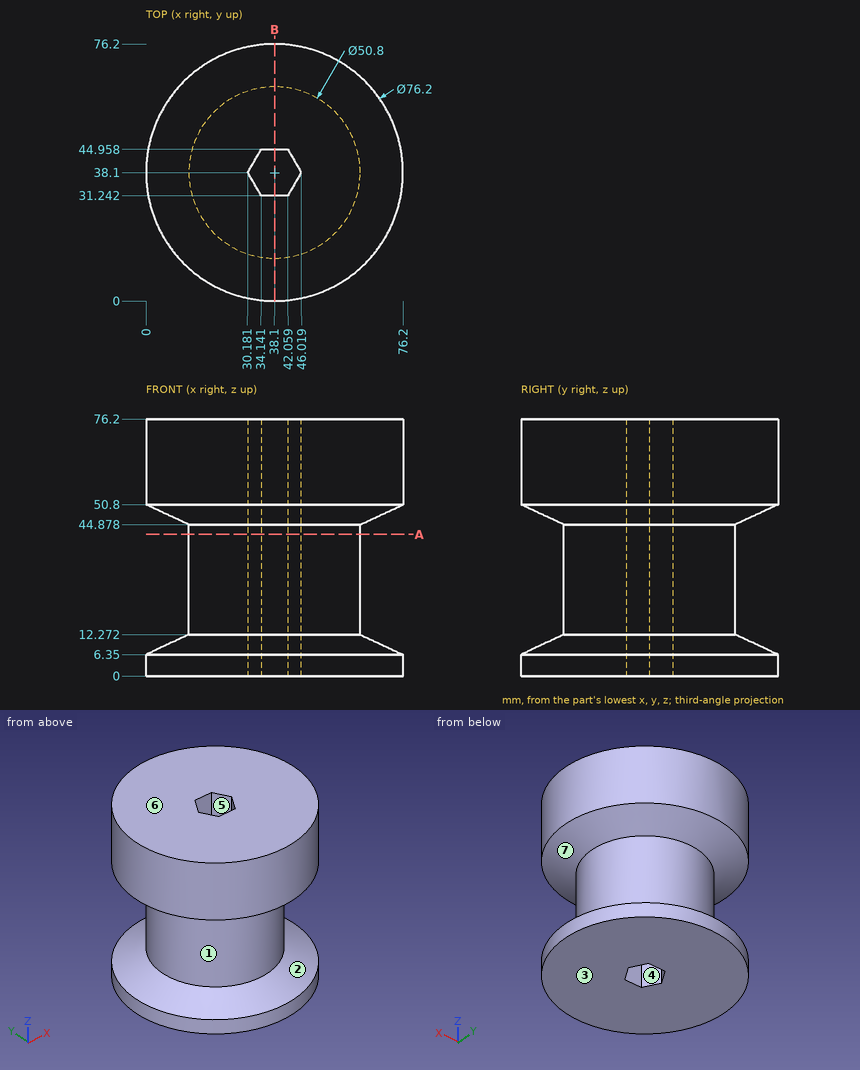
Drawing for the job (mm, zero at the part's lowest x, y, z). A direction names the side the tool comes from. Coordinates: 2 decimals unless noted, no trailing zeros. Order: outer loops, then holes, each group sorted by start corner. A loop starts at its lowest first (then second) coordinate and runs counter-clockwise, first axis right, second up. Notation, with made-up numbers: (17.25, 44) -> (41.25, 44) arc R18 cw to (41.25, 77) -> close; hole circle Ø1 at (28.5, 43). An arc over 180 degrees is marked (long way). One line per item, written item: value.
(1) Tool access for the marked faces 5, 6 and 7: list every direction of +Z, -Z, +X, -X, +Y, -Y with a clear straight run to the whole face (end or side of a thin tool).
Checked values:
face 5: +Z, -Z
face 6: +Z, +X, -X, +Y, -Y
face 7: none
(2) Slice it at B-B, the plane x = 38.1. List the corners of the cut face in (y, z).
Checked values:
outline: (0, 0) -> (31.24, 0) -> (31.24, 76.2) -> (0, 76.2) -> (0, 50.8) -> (12.7, 44.88) -> (12.7, 12.27) -> (0, 6.35) -> close; (44.96, 0) -> (76.2, 0) -> (76.2, 6.35) -> (63.5, 12.27) -> (63.5, 44.88) -> (76.2, 50.8) -> (76.2, 76.2) -> (44.96, 76.2) -> close
(3) Drop flat-ended pins along their axis: pin 1 Ø12 at (x, z) = (48.5, 65) entering from +Y (1 decimal); pin 2 Ø10 at (x, z) = (57.5, 64) entering from +Y (1 decimal); pin 3 Ø3 at (y, z) = (43, 37) entering from -X. Give the stop position or say it passes through.
Checked values:
pin 1: y = 75.9
pin 2: y = 73.4
pin 3: x = 12.93
(4) Probe line 1 (Z direction, x = 20.5, y = 17.5); line 2 (Y direction, x = 37, z = 73.5) (1 decimal); line 3 (Y direction, x = 34, z = 72.5) (1 decimal). List the from-to ranges inside material, lowest first. Write a range as [from, to].
Checked values:
line 1: [0, 11.48], [45.67, 76.2]
line 2: [0, 31.2], [45, 76.2]
line 3: [0.2, 31.5], [44.7, 76]
(5) Slice it at A-A, the plane z = 42. List the corners of the cut face in (x, y).
Checked values:
outline: circle Ø50.8 at (38.1, 38.1); hole (30.18, 38.1) -> (34.14, 31.24) -> (42.06, 31.24) -> (46.02, 38.1) -> (42.06, 44.96) -> (34.14, 44.96) -> close
(6) Mould opens along Z. For the marked faces 1, 2, 3 and 4 say: pulls with the +Z half, pulls with the -Z half, needs draft (parallel to the pull), parting line crosses it, or undercut.
Checked values:
face 1: undercut
face 2: undercut
face 3: pulls with the -Z half
face 4: needs draft
